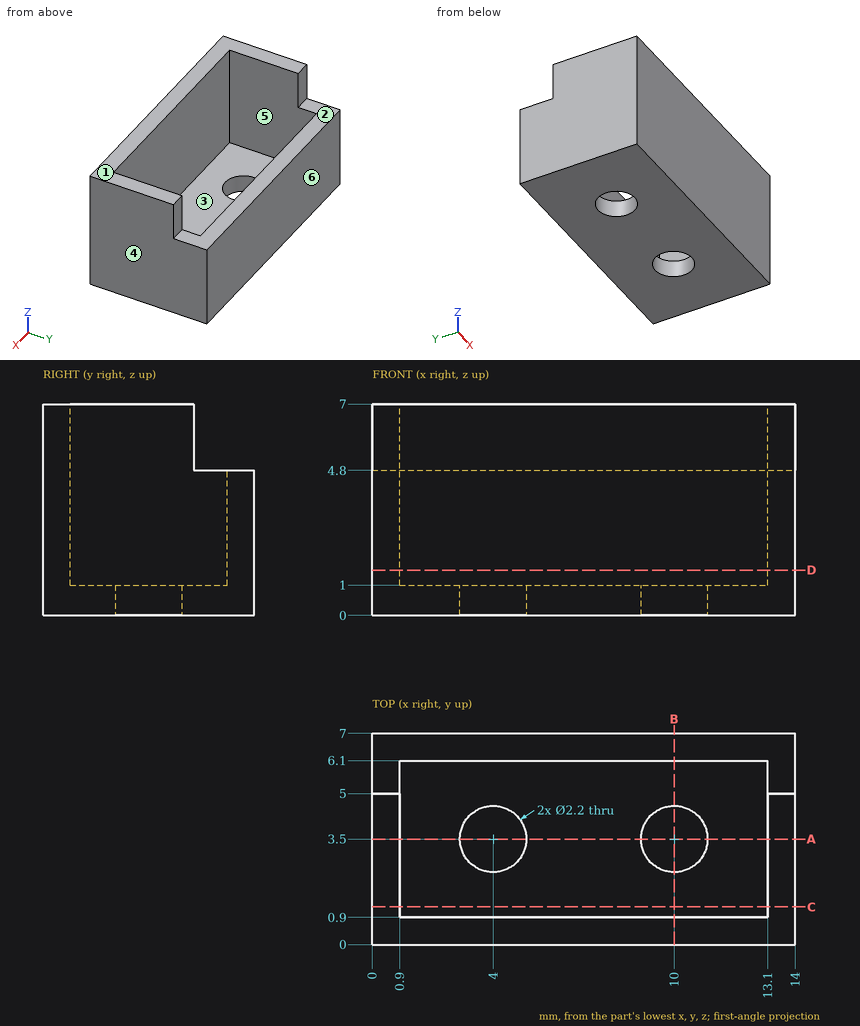
Could you check a few things on this drawing? It's one solid part, dimensions in mm from its lowest x, y, z. A direction names the side the tool comes from. Give positions to 0.01 mm unless a question says otherwise; leave off trailing zeros. Order: outer loops, then holes, each group sorted by start corner. A loop starts at its lowest first (then second) coordinate and runs counter-clockwise, first axis right, second up. Notation, with made-up numbers: (-32.75, 18) - (-12.75, 18) arc R20 ccw to (-12.75, 47) - close; hole circle Ø7 at (44.25, 89.25). An arc over 180 degrees is marked (long way). One line per item, written item: value. Start each with the question number.
1. For P1, Ø3, axis at x = 11, y = 3.5, coming from the +Z side; P2, Ø0.5, axis at x = 0.5, z = 6.5, coming from the +Y side; P3, Ø1.3, axis at x = 10, y = 3.5, coming from the -Z side; P4, Ø1, axis at x = 3.5, y = 6, coming from the +Z side, each with a flat end and sliding along its axis, tell me the tip position at first contact or that it passes through.
2. Imagine slicing it at A-A on y = 3.5. List the corners of the cut face in (x, z) for me, plus the area to 3 significant figures.
3. For the marked faces 1, 2 and 3, which set-ups out of +Z, -Z, +X, -X, +Y, -Y let a thin tool reach every point of the face, with its end or its side?
4. If I drill on probe 1 along Y at (x, z) = (10, 0.7); probe 2 along X at (y, z) = (4.25, 4); probe 3 along Y at (x, z) = (2, 2.5), over which ranges is the centre line in solid material (lowest first)?
5. Imagine slicing it at D-D on z = 1.5. List the corners of the cut face in (x, y) for me, plus the area to 3 significant figures.
6. Thinking about a two-plate mould opening in Y: for the marked faces 4, 5 and 6, which applies, +Y half, -Y half, draft (parallel to the pull), parting line (faces both ways), or undercut?
7. Imagine slicing it at C-C on y = 1.25. List the corners of the cut face in (x, z) for me, plus the area to 3 significant figures.
8. Imagine slicing it at B-B on x = 10. List the corners of the cut face in (y, z) for me.
Values:
1. P1: z = 1
1. P2: y = 5
1. P3: through
1. P4: z = 4.8
2. outline: (0, 0) - (2.9, 0) - (2.9, 1) - (0.9, 1) - (0.9, 7) - (0, 7) - close; (5.1, 0) - (8.9, 0) - (8.9, 1) - (5.1, 1) - close; (11.1, 0) - (14, 0) - (14, 7) - (13.1, 7) - (13.1, 1) - (11.1, 1) - close
2. area: 20.4 mm²
3. face 1: +Z, +X, -X, +Y, -Y
3. face 2: +Z, +X, -X, +Y
3. face 3: +Z
4. probe 1: 0 to 2.4, 4.6 to 7
4. probe 2: 0 to 0.9, 13.1 to 14
4. probe 3: 0 to 0.9, 6.1 to 7
5. outline: (0, 0) - (14, 0) - (14, 7) - (0, 7) - close; hole (0.9, 0.9) - (13.1, 0.9) - (13.1, 6.1) - (0.9, 6.1) - close
5. area: 34.6 mm²
6. face 4: draft
6. face 5: undercut
6. face 6: +Y half
7. outline: (0, 0) - (14, 0) - (14, 7) - (13.1, 7) - (13.1, 1) - (0.9, 1) - (0.9, 7) - (0, 7) - close
7. area: 24.8 mm²
8. outline: (0, 0) - (2.4, 0) - (2.4, 1) - (0.9, 1) - (0.9, 7) - (0, 7) - close; (4.6, 0) - (7, 0) - (7, 4.8) - (6.1, 4.8) - (6.1, 1) - (4.6, 1) - close
